Design review of the part built by this model. Coordinates are the model's own, in mm. Face numbers are marked on the shaded views. Give positions to 0.01 mm unless a question says otherwise; leave off trailing zeros. Order: outer loops, then holes, each group sorted by start corner. A loop starts at its lowest first (then second) coordinate and runs counter-clockwise, first axis right, second up. Notation, with made-up numbers: (72.25, 54.25) -> (108.25, 54.25) arc R20 cw to (108.25, 78.25) -> close; hole circle Ø6 at (35, 11.25). An arc over 180 degrees is marked (long way). One line per item, written item: value.
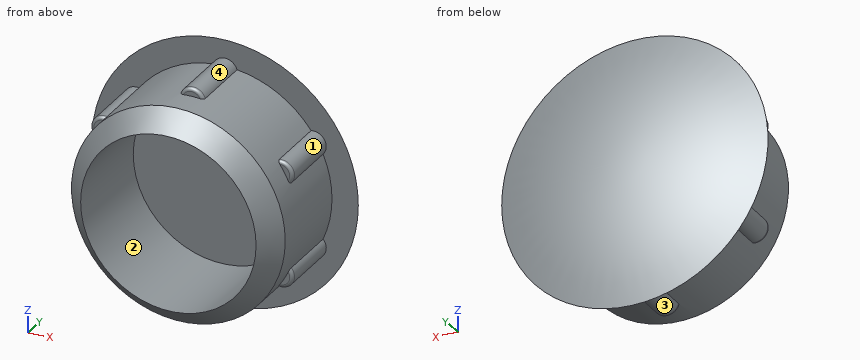
from build123d import *

# Parameters (mm, degrees)
EXTRUDE_1_DEPTH          = 4
PATTERN_CIRCULAR_1_COUNT = 6
FILLET_1_R               = 0.2


with BuildPart() as part:
    # Эскиз1 → Повернуть1 (revolve)
    with BuildSketch(Plane.XY):
        with BuildLine():
            Line((8.35, 0), (6.7, 0))
            Line((6.7, 0), (6.7, -5.6))
            Line((6.7, -5.6), (5.5, -6.8))
            Line((5.5, -6.8), (5.5, -0.5))
            Line((5.5, -0.5), (0, -0.5))
            Line((0, -0.5), (0, 1.5))
            ThreePointArc((0, 1.5), (4.241830383, 1.122022467), (8.35, 0))
        make_face()
    revolve(axis=Axis((0, -0.5, 0), (0, -1, 0)))

    # Эскиз2 → Бобышка-Вытянуть1 (add)
    with BuildSketch(Plane.XZ):
        with BuildLine():
            ThreePointArc((-0.75, 6.657890056), (0, 7.2), (0.75, 6.657890056))
            ThreePointArc((0.75, 6.657890056), (0, 6.7), (-0.75, 6.657890056))
        make_face()
    extrude_1 = extrude(amount=EXTRUDE_1_DEPTH)

    # Круговой массив1: Бобышка-Вытянуть1 ×6 about axis
    pattern_circular_1_axis = Axis((0, 0, 0), (0, 1, 0))
    for i in range(1, PATTERN_CIRCULAR_1_COUNT):
        add(extrude_1.rotate(pattern_circular_1_axis, i * 360 / PATTERN_CIRCULAR_1_COUNT))

    # Скругление1
    fillet_1_edges = [part.edges().sort_by_distance(p)[0] for p in [
        (0, -4, 7.2),
        (6.235382907, -4, 3.6),
        (6.235382907, -4, -3.6),
        (0, -4, -7.2),
        (-6.235382907, -4, -3.6),
        (-6.235382907, -4, 3.6),
    ]]
    fillet(fillet_1_edges, radius=FILLET_1_R)


solid = part.part
Item 1: Draft analysis for pull direction Z (two halves, no side actions). For the marked faces 1, 2, 3 and 4, state which applies: pulls with the +Z half, pulls with the -Z half, needs draft (parallel to the pull), parting line crosses it, or undercut.
Returned:
face 1: undercut
face 2: undercut
face 3: pulls with the -Z half
face 4: pulls with the +Z half
Item 2: Clearance check with flat-ended pins moving along their axes: P1, Ø1, axis at x = 1, z = 1.5, coming from the -Y side; P2, Ø5, axis at x = 4.5, z = 0.5, coming from the +Y side; P3, Ø1, axis at y = -4, z = 5.5, coming from the -X side. State where each tip first meets the part, or that it passes through.
Returned:
P1: y = -0.5
P2: y = 1.41
P3: x = -4.46
Item 3: Add section A-A on x = 0. Give the boundary of the cut face in (y, z).
Returned:
outline: (-6.8, -5.5) -> (-5.6, -6.7) -> (-4, -6.7) -> (-4, -7) arc R0.2 ccw to (-3.8, -7.2) -> (0, -7.2) -> (0, -8.35) arc R23.99 ccw to (0, 8.35) -> (0, 7.2) -> (-3.8, 7.2) arc R0.2 ccw to (-4, 7) -> (-4, 6.7) -> (-5.6, 6.7) -> (-6.8, 5.5) -> (-0.5, 5.5) -> (-0.5, -5.5) -> close
Item 4: Add section B-B on z = 0. Give the boundary of the cut face in (x, y).
Returned:
outline: (-8.35, 0) -> (-6.7, 0) -> (-6.7, -5.6) -> (-5.5, -6.8) -> (-5.5, -0.5) -> (5.5, -0.5) -> (5.5, -6.8) -> (6.7, -5.6) -> (6.7, 0) -> (8.35, 0) arc R23.99 ccw to start
Item 5: To check wall thickness, follow line 1 along Z through (x, y) = (0, -5.25); line 2 along Z through (x, y) = (-3.75, -3); line 3 along X through (y, z) = (-0.75, -1.5). State the ranges of each line that lie inside material, in increasing order. Write a range as from..to.
Returned:
line 1: -6.7..-5.5, 5.5..6.7
line 2: -5.55..-4.02, 4.02..5.55
line 3: -6.53..-5.29, 5.29..6.53
Item 6: Add section D-D on y = -6. Give the boundary of the cut face in (x, z).
Returned:
outline: circle Ø12.6 at (0, 0); hole circle Ø11 at (0, 0)
Item 7: Add section C-C on y = -2.75. Give the boundary of the cut face in (x, z).
Returned:
outline: (-6.14, -2.68) arc R0.79 ccw to (-5.39, -3.98) arc R6.7 ccw to (-0.75, -6.66) arc R0.79 ccw to (0.75, -6.66) arc R6.7 ccw to (5.39, -3.98) arc R0.79 ccw to (6.14, -2.68) arc R6.7 ccw to (6.14, 2.68) arc R0.79 ccw to (5.39, 3.98) arc R6.7 ccw to (0.75, 6.66) arc R0.79 ccw to (-0.75, 6.66) arc R6.7 ccw to (-5.39, 3.98) arc R0.79 ccw to (-6.14, 2.68) arc R6.7 ccw to start; hole circle Ø11 at (0, 0)
